Can you work these out from the model? Positions are in its coordinate system, mm. Face numbers are marked on the shaded views. A direction names the side the tool comes from. Round coordinates to 2 decimals unless told otherwise and drop trailing zeros. Loops run counter-clockwise (first coordinate to the right, second up) from the corner with the lowest first, then second, coordinate; pieces in that order, holes last.
(1) If I drill on line 1 along X through (y, z) = (-1, -1); line 2 along X through (y, z) = (-3.75, -2.25); line 3 along Z through (x, y) = (27.5, 2), over which ranges is the centre line in solid material (lowest first)?
(2) Will these pins go through, and if not, where does the flat tip stop? pin 1 Ø0.5 at (x, y) = (2, 0.5) entering from -Z; pin 2 Ø4 at (x, z) = (9.5, 2) entering from -Y; pin 3 Ø2 at (x, z) = (17.5, 0.5) entering from +Y.
(3) Thinking about a two-plate mould opening in Z: for the marked faces 4, 5 and 6, which applies, released by +Z, released by -Z, zero draft, split by the parting line, or undercut?
(4) Which directions (+Z, -Z, +X, -X, +Y, -Y) give clear straight access to the entire face, cutting with the end or side of a thin tool? Please do the marked faces 1, 2 and 3.
(5) I want a section at C-C on z = 3.5. Write out the boundary of the cut face in (x, y), plus the area to 3 significant figures.
(6) I want a section at A-A on y = 0. Write out the boundary of the cut face in (x, z), plus the area to 3 significant figures.
(7) I want a section at B-B on x = 17.5. Write out the boundary of the cut face in (y, z).
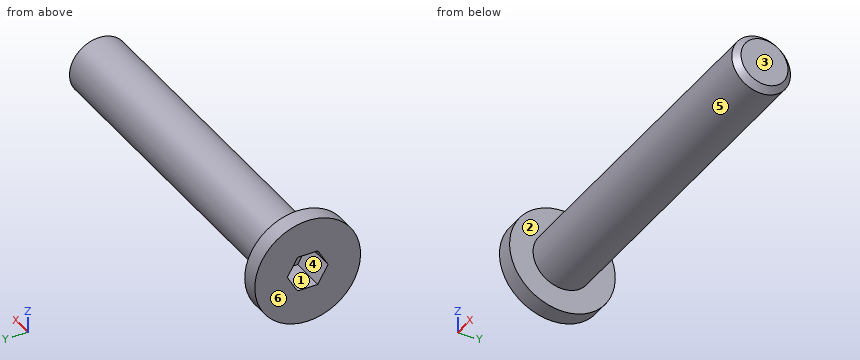
from build123d import *

# Parameters (mm, degrees)
SKETCH1_R     = 4.5
HEAD_DEPTH    = 1.5
SKETCH2_R     = 2.5
BODY_DEPTH    = 30
DRIVE_DEPTH   = 3
CHAMFER1_SIZE = 0.5


with BuildPart() as part:
    # Sketch1 → Head (new body)
    with BuildSketch(Plane(origin=(0, 0, 0), x_dir=(0, 0, -1), z_dir=(1, 0, 0))):
        Circle(SKETCH1_R)
    extrude(amount=HEAD_DEPTH)

    # Sketch2 → Body (add)
    with BuildSketch(Plane(origin=(1.5, 0, 0), x_dir=(0, 0, -1), z_dir=(1, 0, 0))):
        Circle(SKETCH2_R)
    extrude(amount=BODY_DEPTH)

    # Sketch3 → Drive (cut)
    with BuildSketch(Plane.ZY):
        Polygon((0, 1.732050808), (-1.5, 0.866025404), (-1.5, -0.866025404), (0, -1.732050808), (1.5, -0.866025404), (1.5, 0.866025404), align=None)
    extrude(amount=-DRIVE_DEPTH, mode=Mode.SUBTRACT)

    # Chamfer1
    chamfer1_edges = [part.edges().sort_by_distance(p)[0] for p in [
        (31.5, 0, 2.5),
    ]]
    chamfer(chamfer1_edges, length=CHAMFER1_SIZE)


solid = part.part
Filled sheet:
1. line 1: x = 3 to 31.5
1. line 2: x = 0 to 1.5
1. line 3: z = -1.5 to 1.5
2. pin 1: stops at z = -2.49
2. pin 2: stops at y = -2.5
2. pin 3: stops at y = 2.5
3. face 4: undercut
3. face 5: split by the parting line
3. face 6: zero draft
4. face 1: -X
4. face 2: +X
4. face 3: +Z, -Z, +X, +Y, -Y
5. outline: (0, -2.83) - (1.5, -2.83) - (1.5, 2.83) - (0, 2.83) - close
5. area: 8.49 mm2
6. outline: (0, -4.5) - (1.5, -4.5) - (1.5, -2.5) - (31, -2.5) - (31.5, -2) - (31.5, 2) - (31, 2.5) - (1.5, 2.5) - (1.5, 4.5) - (0, 4.5) - (0, 1.5) - (3, 1.5) - (3, -1.5) - (0, -1.5) - close
6. area: 154 mm2
7. outline: circle Ø5 at (0, 0)
